from build123d import *

# Parameters (mm, degrees)
F0_R     = 11.049
F1_DEPTH = 6.35
F2_R     = 2.54
F3_R     = 2.54


with BuildPart() as f1:
    # F0 (on Top) → F1 (new body)
    with BuildSketch(Plane.XY):
        with BuildLine():
            ThreePointArc((-12.098375, 23.495), (-9.886454, 15.24), (-12.098375, 6.985))
            ThreePointArc((-12.098375, 6.985), (0, -13.97), (12.098375, 6.985))
            ThreePointArc((12.098375, 6.985), (9.886454, 15.24), (12.098375, 23.495))
            ThreePointArc((12.098375, 23.495), (0, 44.45), (-12.098375, 23.495))
        make_face()
        Circle(F0_R, mode=Mode.SUBTRACT)
        with Locations((0, 30.48)):
            Circle(F0_R, mode=Mode.SUBTRACT)
    extrude(amount=F1_DEPTH)

    # F2
    f2_edges = [f1.edges().sort_by_distance(p)[0] for p in [
        (0, -13.97, 6.35),
    ]]
    fillet(f2_edges, radius=F2_R)

    # F3
    f3_edges = [f1.edges().sort_by_distance(p)[0] for p in [
        (0, -13.97, 0),
    ]]
    fillet(f3_edges, radius=F3_R)


solid = f1.part
Read the model definition and answer for the solid it produces. Units are mm, in the model's axes. Coordinates: 2 decimals unless noted, no trailing zeros. Order: outer loops, then holes, each group sorted by start corner. A loop starts at its lowest first (then second) coordinate and runs counter-clockwise, first axis right, second up. Notation, with made-up numbers: M -4,80.5 L 15,80.5 A22 cw 15,105.5 Z; hole C 14.5,41.25 d7. An arc over 180 degrees is marked long. Put each result on its own line as item: value. Start each with the question number.
Item 1: Given pin 1 Ø6 at (x, y) = (-5, 35) entering from -Z; pin 2 Ø1 at (y, z) = (37, 4) entering from +X; pin 3 Ø1.5 at (x, z) = (-10.5, 2.5) entering from -Y; pin 4 Ø1.5 at (x, z) = (4, 5) entering from +Y, each flat-ended and moving along its own axis, determine where each tip first touches the part or whether it passes through.
Item 2: The mould has two halves that part along Y. Classify faces 1 (the face through (0, 15, 6.35)), 2 (the face through (-0.41, -13.964, 3.166)): +Y half, -Y half, draft (parallel to the pull), parting line (faces both ways), or undercut.
Item 3: Consider probe 1 along Y at (x, z) = (0.25, 3.5); probe 2 along Y at (x, z) = (3.5, 3.75); probe 3 along X at (y, z) = (33.5, 4.5). Determine where each line is inside the solid, lowest interval first. Write a range as [from, to].
Item 4: Section B-B, the plane z = 3.25 is taken. Determine the outline of the cut face in (x, y) (3 decimals), plus the area to 3 significant figures.
Item 5: Section A-A, the plane x = 0 is taken. Determine the outline of the cut face in (y, z), plus the area to 3 significant figures.
Item 6: Section C-C, the plane x = -6 is taken. Count the separate pieces of the cut face and the enclosed holes in it, plus the area to 3 significant figures.
Computed:
1. pin 1: passes through
1. pin 2: stops at x = 12.6
1. pin 3: stops at y = -10
1. pin 4: stops at y = 43.92
2. face 1: draft
2. face 2: undercut
3. probe 1: y = [-13.97, -11.05], [11.05, 19.43], [41.53, 44.45]
3. probe 2: y = [-13.52, -10.48], [10.48, 20], [40.96, 44]
3. probe 3: x = [-13.54, -10.63], [10.63, 13.54]
4. outline: M -12.098,6.985 A13.97 ccw long 12.098,6.985 A16.51 cw 12.098,23.495 A13.97 ccw long -12.098,23.495 A16.51 cw Z; hole C 0,0 d22.098; hole C 0,30.48 d22.098
4. area: 570 mm2
5. outline: M -13.97,2.54 A2.54 ccw -11.43,0 L -11.05,0 L -11.05,6.35 L -11.43,6.35 A2.54 ccw -13.97,3.81 Z; M 11.05,0 L 19.43,0 L 19.43,6.35 L 11.05,6.35 Z; M 41.53,0 L 41.91,0 A2.54 ccw 44.45,2.54 L 44.45,3.81 A2.54 ccw 41.91,6.35 L 41.53,6.35 Z
5. area: 84.8 mm2
6. separate pieces: 3
6. enclosed holes: 0
6. area: 112 mm2
